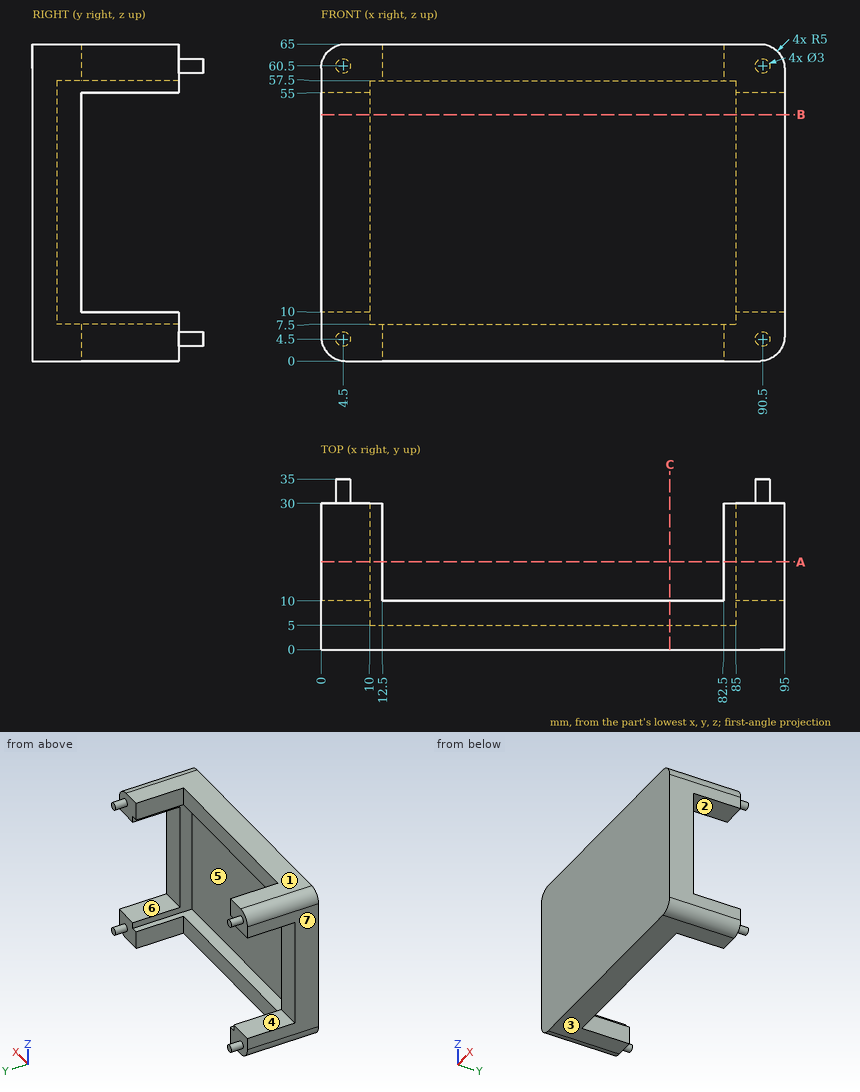
Can you work these out from the drawing? Everything is in mm from the part's minimum corner. A direction names the side the tool comes from. Give positions to 0.01 mm unless a question says otherwise; leave off trailing zeros. Loops run counter-clockwise (first coordinate to the right, second up) from the corner with the lowest first, then second, coordinate; pieces in that order, holes last. Notation, with made-up numbers: M 18,29.5 L 73,29.5 A24 ccw 73,42.5 Z; hole C -3.5,-8 d4. An arc over 180 degrees is marked long. Put each result on its own line as item: value. Start each with the question number.
(1) Will these pins go through, and if not, where does the flat tip stop? pin 1 Ø6 at (y, z) = (24, 4) entering from +X; pin 2 Ø4 at (x, z) = (42.5, 59.5) entering from +Y; pin 3 Ø3 at (x, y) = (3, 19) entering from -Z; pin 4 Ø10 at (x, z) = (23.5, 49) entering from +Y.
(2) I want a section at C-C on x = 71.5. Please give me the cut outline in (y, z), then the cut area to 3 significant figures.
(3) For the marked faces 5, 6 and 7, which set-ups out of +Z, -Z, +X, -X, +Y, -Y let a thin tool reach every point of the face, with its end or its side?
(4) I want a section at B-B on z = 50.5. Please give me the cut outline in (x, y), then the cut area to 3 significant figures.
(5) If we mould it in two halves opening along Z, with no side actions, what happens to the marked faces 1, 2, 3 and 4? For each: +Z half, -Z half, draft (parallel to the pull), parting line (faces both ways), or undercut.
(6) I want a section at A-A on y = 18. Please give me the cut outline in (x, z), then the cut area to 3 significant figures.
(7) I need wall thicknesses on line 1 along Z through (x, y) = (36, 6); line 2 along X through (y, z) = (6.5, 13.5); line 3 along Z through (x, y) = (86.5, 14.5). Which ranges of each line are inside material? Lowest first, please. Write a range as [from, to].
Answer block:
1. pin 1: x = 95
1. pin 2: y = 10
1. pin 3: z = 0.03
1. pin 4: y = 5
2. outline: M 0,0 L 10,0 L 10,7.5 L 5,7.5 L 5,57.5 L 10,57.5 L 10,65 L 0,65 Z
2. area: 400 mm^2
3. face 5: +Y
3. face 6: +X, -X, +Y
3. face 7: +Z, -Z, -X, +Y, -Y
4. outline: M 0,0 L 95,0 L 95,10 L 85,10 L 85,5 L 10,5 L 10,10 L 0,10 Z
4. area: 575 mm^2
5. face 1: +Z half
5. face 2: undercut
5. face 3: -Z half
5. face 4: undercut
6. outline: M 0,5 A5 ccw 5,0 L 12.5,0 L 12.5,7.5 L 10,7.5 L 10,10 L 0,10 Z; M 0,55 L 10,55 L 10,57.5 L 12.5,57.5 L 12.5,65 L 5,65 A5 ccw 0,60 Z; M 82.5,0 L 90,0 A5 ccw 95,5 L 95,10 L 85,10 L 85,7.5 L 82.5,7.5 Z; M 82.5,57.5 L 85,57.5 L 85,55 L 95,55 L 95,60 A5 ccw 90,65 L 82.5,65 Z
6. area: 454 mm^2
7. line 1: [0, 7.5], [57.5, 65]
7. line 2: [0, 10], [85, 95]
7. line 3: [0, 10], [55, 65]
